```python
from build123d import *

# Parameters (mm, degrees)
SKETCH1_W           = 80
SKETCH1_H           = 100
BOSS_EXTRUDE1_DEPTH = 12.5
CUT_EXTRUDE1_DEPTH  = 5
CUT_EXTRUDE4_START  = 5
CUT_EXTRUDE4_DEPTH  = 5


with BuildPart() as part:
    # Sketch1 → Boss-Extrude1 (new body)
    with BuildSketch(Plane(origin=(0, 0, 0), x_dir=(1, 0, 0), z_dir=(0, 1, 0))):
        with Locations((40, 50)):
            Rectangle(SKETCH1_W, SKETCH1_H)
    extrude(amount=BOSS_EXTRUDE1_DEPTH)

    # Sketch2 → Cut-Extrude1 (cut)
    with BuildSketch(Plane.XY):
        with BuildLine():
            ThreePointArc((73, 2.895898034), (76.091650066, 3.44375696), (77.5, 6.25))
            Line((77.5, 6.25), (74, 6.25))
            Line((74, 6.25), (73, 6.25))
            Line((73, 6.25), (73, 2.895898034))
        make_face()
        with BuildLine():
            Line((74, 6.25), (77.5, 6.25))
            ThreePointArc((77.5, 6.25), (76.091650066, 9.05624304), (73, 9.604101966))
            Line((73, 9.604101966), (73, 6.25))
            Line((73, 6.25), (74, 6.25))
        make_face()
        with BuildLine():
            Line((73, 6.25), (73, 9.604101966))
            ThreePointArc((73, 9.604101966), (71.19375696, 8.341650066), (70.5, 6.25))
            Line((70.5, 6.25), (73, 6.25))
        make_face()
        with BuildLine():
            ThreePointArc((70.5, 6.25), (71.19375696, 4.158349934), (73, 2.895898034))
            Line((73, 2.895898034), (73, 6.25))
            Line((73, 6.25), (70.5, 6.25))
        make_face()
        with BuildLine():
            ThreePointArc((59.5, 5.25), (66.307499895, 4.402691993), (73, 2.895898034))
            ThreePointArc((73, 2.895898034), (71.19375696, 4.158349934), (70.5, 6.25))
            Line((70.5, 6.25), (59.5, 6.25))
            Line((59.5, 6.25), (58.5, 6.25))
            ThreePointArc((58.5, 6.25), (58.814539324, 5.564539324), (59.5, 5.25))
        make_face()
        with BuildLine():
            ThreePointArc((70.5, 6.25), (71.19375696, 8.341650066), (73, 9.604101966))
            ThreePointArc((73, 9.604101966), (66.311170081, 8.076260701), (59.5, 7.25))
            ThreePointArc((59.5, 7.25), (58.812768212, 6.937231788), (58.5, 6.25))
            Line((58.5, 6.25), (59.5, 6.25))
            Line((59.5, 6.25), (70.5, 6.25))
        make_face()
    extrude(amount=-CUT_EXTRUDE1_DEPTH, mode=Mode.SUBTRACT)

    # Sketch6 → Cut-Extrude4 (cut)
    with BuildSketch(Plane.XY.offset(-100).offset(CUT_EXTRUDE4_START)):
        with BuildLine():
            ThreePointArc((73, 2.895898034), (77.5, 6.25), (73, 9.604101966))
            ThreePointArc((73, 9.604101966), (66.352079757, 7.840991059), (59.499996599, 7.247391846))
            ThreePointArc((59.499996599, 7.247391846), (58.499996599, 6.247391846), (59.499996599, 5.247391846))
            ThreePointArc((59.499996599, 5.247391846), (66.351631714, 4.655125717), (73, 2.895898034))
        make_face()
    extrude(amount=-CUT_EXTRUDE4_DEPTH, mode=Mode.SUBTRACT)


solid = part.part
```
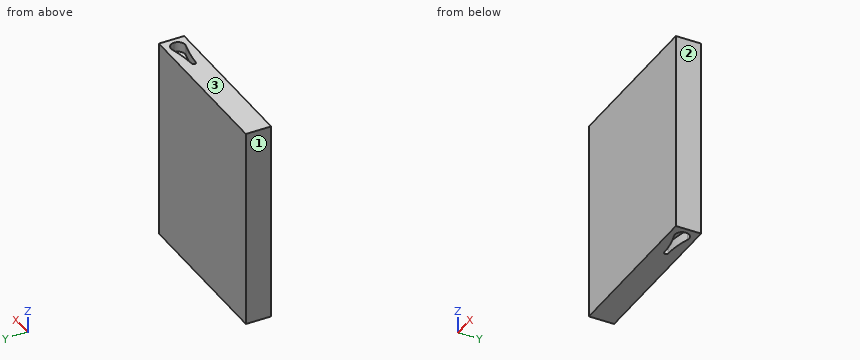
Here's how the part is built. I have some questions about the finished solid (model axes, mm). Face numbers are marked on the shaded views. Coordinates: 2 decimals unless noted, no trailing zeros. Return JSON: item names as keys, results as strings. Group by question number.
Item 1: Will this pin go through, and if not, where does the flat tip stop? P1, Ø2, axis at x = 69.5, y = 6.5, coming from the +Z side.
Item 2: We'd pull the mould along X, two halves only. Please class the marked faces 1, 2 and 3: +X half, -X half, draft (parallel to the pull), parting line (faces both ways), or undercut.
Item 3: I need wall thicknesses on line 1 (Y direction, x = 74, z = -99); line 2 (X direction, y = 6.25, z = -96.7); line 3 (Z direction, x = 61.5, y = 6.5). Which ranges of each line are inside material? Lowest first, please. Write a range as from..to.
Calculated:
{
 "1": {"P1": "stops at z = -5"},
 "2": {"face 1": "-X half", "face 2": "+X half", "face 3": "draft"},
 "3": {"line 1": "y = 0..2.75, 9.75..12.5", "line 2": "x = 0..58.5, 77.5..80", "line 3": "z = -95..-5"}
}
